CAD build for the part. Positions are in the model's coordinates, mm. Coordinates: 2 decimals unless noted, no trailing zeros. Loops run counter-clockwise (first coordinate to the right, second up) from the corner with the lowest first, then second, coordinate; pieces in that order, holes last. Notation, with made-up numbers: (54, 10.5) -> (85, 10.5) arc R26 cw to (85, 49.5) -> close; hole circle Ø4 at (55, 89). An arc over 180 degrees is marked (long way). Answer as CSV lines item,"result". Start each with the question number.
from build123d import *

# Parameters (mm, degrees)
SKETCH1_W           = 40
SKETCH1_H           = 8
SKETCH1_R           = 2.1
SKETCH1_R_2         = 1.25
BOSS_EXTRUDE1_DEPTH = 8
SKETCH2_R           = 1.25
CUT_EXTRUDE1_DEPTH  = 9


with BuildPart() as part:
    # Sketch1 → Boss-Extrude1 (new body)
    with BuildSketch(Plane.XY):
        Rectangle(SKETCH1_W, SKETCH1_H)
        Circle(SKETCH1_R, mode=Mode.SUBTRACT)
        with Locations((7.5, 0)):
            Circle(SKETCH1_R_2, mode=Mode.SUBTRACT)
        with Locations((-7.5, 0)):
            Circle(SKETCH1_R_2, mode=Mode.SUBTRACT)
    extrude(amount=BOSS_EXTRUDE1_DEPTH)

    # Sketch2 → Cut-Extrude1 (cut, through all)
    with BuildSketch(Plane.XZ.offset(4)):
        with Locations((-16, 4)):
            Circle(SKETCH2_R)
        with Locations((16, 4)):
            Circle(SKETCH2_R)
    extrude(amount=-CUT_EXTRUDE1_DEPTH, mode=Mode.SUBTRACT)


solid = part.part
Item 1: Saw through at C-C (x = -16). Write the cut outline in (y, z).
Item 2: Saw through at D-D (y = -2.75). Write the cut outline in (x, z), plus the area to 3 significant figures.
Item 3: Two-plate mould, pull along Y, no slides. Class faces 1 (the face through (6.25, 0.05, 3.94)), 2 (the face through (0, 3, 0)), 3 (the face through (0, 4, 4)): pulls with the +Y half, pulls with the -Y half, needs draft (parallel to the pull), parting line crosses it, or undercut.
Item 4: Saw through at A-A (y = 0). Write the cut outline in (x, z).
Item 5: Wall check: probe 1 along Z at (x, y) = (16, 1.25); probe 2 along X at (y, z) = (0.5, 1.75); probe 3 along Y at (x, z) = (0, 4). Give the ranges that are in metal, low to high.
Item 6: Saw through at B-B (z = 4). Write the cut outline in (x, y), plus the area to 3 significant figures.
Geometry check:
1,outline,"(-4, 0) -> (4, 0) -> (4, 2.75) -> (-4, 2.75) -> close; (-4, 5.25) -> (4, 5.25) -> (4, 8) -> (-4, 8) -> close"
2,outline,"(-20, 0) -> (20, 0) -> (20, 8) -> (-20, 8) -> close; hole circle Ø2.5 at (-16, 4); hole circle Ø2.5 at (16, 4)"
2,area,"310 mm2"
3,face 1,"undercut"
3,face 2,"needs draft"
3,face 3,"pulls with the +Y half"
4,outline,"(-20, 0) -> (-8.75, 0) -> (-8.75, 8) -> (-20, 8) -> close; (-6.25, 0) -> (-2.1, 0) -> (-2.1, 8) -> (-6.25, 8) -> close; (2.1, 0) -> (6.25, 0) -> (6.25, 8) -> (2.1, 8) -> close; (8.75, 0) -> (20, 0) -> (20, 8) -> (8.75, 8) -> close; hole circle Ø2.5 at (-16, 4); hole circle Ø2.5 at (16, 4)"
5,probe 1,"0 to 2.75, 5.25 to 8"
5,probe 2,"-20 to -8.65, -6.35 to -2.04, 2.04 to 6.35, 8.65 to 20"
5,probe 3,"-4 to -2.1, 2.1 to 4"
6,outline,"(-20, -4) -> (-17.25, -4) -> (-17.25, 4) -> (-20, 4) -> close; (-14.75, -4) -> (14.75, -4) -> (14.75, 4) -> (-14.75, 4) -> close; (17.25, -4) -> (20, -4) -> (20, 4) -> (17.25, 4) -> close; hole circle Ø2.5 at (-7.5, 0); hole circle Ø4.2 at (0, 0); hole circle Ø2.5 at (7.5, 0)"
6,area,"256 mm2"
